The listing builds one solid part. Answer for the finished solid, in the listing's coordinates (mm). A direction names the side the tool comes from. Coordinates: 2 decimals unless noted, no trailing zeros. Order: outer loops, then holes, each group sorted by start corner. A loop starts at its lowest first (then second) coordinate and runs counter-clockwise, first axis right, second up. Notation, with made-up numbers: M -6.5,-37.5 L 10.5,-37.5 A23 ccw 10.5,-21.5 Z; hole C 41,35.25 d6. An arc over 180 degrees is marked long. One line per item, written item: value. Start each with the question number.
Q1. For faces 1 (the flat face through (0, 19, 31.5)), 2 (the flat face through (0, 0, 1)), 3 (the flat face through (5.4, 5, 18.9)), determine the directions among +Z, -Z, +X, -X, +Y, -Y from which every point of the face is accessible in a straight line to the end or side of a thin tool.
Q2. Determine the mould class of faces 4 (the flat face through (6, 9, -11.839)), 5 (the flat face through (-7.5, 9, 19)), 6 (the cylindrical face through (-3.97, 2.46, 15.08)), 7 (the cylindrical face through (-0.65, 2.46, -13.16)) for opening direction X: pulls with the +X half, pulls with the -X half, needs draft (parallel to the pull), parting line crosses it, or undercut.
Q3. The part is cut by section C-C on x = -13. Give the vertices of the cut face in (y, z).
Q4. Straight lines are drawn through the part: line 1 along Z through (x, y) = (-7, 5.5); line 2 along Z through (x, y) = (0, 2.65); line 3 along Z through (x, y) = (7, 21). For each, find the intervals that lie inside material, in ascending order. Write a range as [from, to].
Q5. Each of these flat-tipped pins is pushed along its axis until it touches: pin 1 Ø6 at (x, z) = (0, -18.12) entering from -Y; pin 2 Ø4 at (x, z) = (10.5, 19) entering from +Y; pin 3 Ø2.5 at (y, z) = (8.5, -15.5) entering from +X; pin 4 Ø4 at (x, z) = (-7, 5.5) entering from +Y. Where does it stop, or does it pass through?
Q6. The part is cut by section D-D on z = -25. Give the vertices of the cut face in (x, y).
Q7. The part is cut by section A-A on x = 0. Give the vertices of the cut face in (y, z), then the cut area to 3 significant figures.
Q8. The part is cut by section B-B on y = 17.5. Give the vertices of the cut face in (x, z).
```python
from build123d import *

# Parameters (mm, degrees)
F0_W      = 37.5
F0_H      = 63
F3_DEPTH  = 5
F5_DEPTH  = 8
F6_W      = 37.5
F6_H      = 5
F7_DEPTH  = 25
F8_W      = 37.5
F8_H      = 5
F9_DEPTH  = 25
F1_R      = 5
F10_DEPTH = 5


with BuildPart() as f3:
    # F0 (on Front) → F3 (new body)
    with BuildSketch(Plane.XZ):
        Rectangle(F0_W, F0_H)
    extrude(amount=-F3_DEPTH)

    # F4 (on face) → F5 (join)
    with BuildSketch(Plane(origin=(0, 5, 0), x_dir=(-1, 0, 0), z_dir=(0, 1, 0))):
        Polygon((7.5, 11.838892), (0, 11.838892), (-18.75, 11.838892), (-18.75, -11.838892), (0, -11.838892), (7.5, -11.838892), (7.5, -25.838892), (0, -25.838892), (-18.75, -25.838892), (-18.75, -31.5), (18.75, -31.5), (18.75, 31.5), (-18.75, 31.5), (-18.75, 25.838892), (0, 25.838892), (7.5, 25.838892), align=None)
    extrude(amount=F5_DEPTH)

    # F6 (on Front) → F7 (join)
    with BuildSketch(Plane.XZ):
        with Locations((0, 34)):
            Rectangle(F6_W, F6_H)
    extrude(amount=-F7_DEPTH)

    # F8 (on Front) → F9 (join)
    with BuildSketch(Plane.XZ):
        with Locations((0, -34)):
            Rectangle(F8_W, F8_H)
    extrude(amount=-F9_DEPTH)

    # F1 (on face) → F10 (cut)
    with BuildSketch(Plane.XZ):
        with Locations((0, 18.117641)):
            Circle(F1_R)
        with Locations((0, -18.117641)):
            Circle(F1_R)
    extrude(amount=-F10_DEPTH, mode=Mode.SUBTRACT)


solid = f3.part
```
Output:
1. face 1: +X, -X, +Y
1. face 2: +Z, -Z, +X, -X, -Y
1. face 3: +X, +Y
2. face 4: needs draft
2. face 5: pulls with the +X half
2. face 6: undercut
2. face 7: undercut
3. outline: M 0,-36.5 L 25,-36.5 L 25,-31.5 L 13,-31.5 L 13,31.5 L 25,31.5 L 25,36.5 L 0,36.5 Z
4. line 1: z = [-36.5, -25.84], [-11.84, 11.84], [25.84, 36.5]
4. line 2: z = [-36.5, -23.12], [-13.12, 13.12], [23.12, 36.5]
4. line 3: z = [-36.5, -31.5], [31.5, 36.5]
5. pin 1: passes through
5. pin 2: stops at y = 5
5. pin 3: stops at x = -7.5
5. pin 4: stops at y = 13
6. outline: M -18.75,0 L 18.75,0 L 18.75,5 L -7.5,5 L -7.5,13 L -18.75,13 Z
7. outline: M 0,-36.5 L 25,-36.5 L 25,-31.5 L 13,-31.5 L 13,-25.84 L 5,-25.84 L 5,-23.12 L 0,-23.12 Z; M 0,-13.12 L 5,-13.12 L 5,-11.84 L 13,-11.84 L 13,11.84 L 5,11.84 L 5,13.12 L 0,13.12 Z; M 0,23.12 L 5,23.12 L 5,25.84 L 13,25.84 L 13,31.5 L 25,31.5 L 25,36.5 L 0,36.5 Z
7. area: 745 mm^2
8. outline: M -18.75,-36.5 L 18.75,-36.5 L 18.75,-31.5 L -18.75,-31.5 Z; M -18.75,31.5 L 18.75,31.5 L 18.75,36.5 L -18.75,36.5 Z
